Job drawing, mm, ordinate dimensions from the low corner. One solid piece. Round coordinates to 2 decimals unless told otherwise and drop trailing zeros. Loops run counter-clockwise (first coordinate to the right, second up) from the corner with the lowest first, then second, coordinate; pieces in that order, holes last. Notation, with made-up numbers: M 81,-37 L 90,-37 A19 cw 90,-3 Z; hole C -5.75,-11.75 d4. An arc over 180 degrees is marked long. Use one line per item in the form item = value.
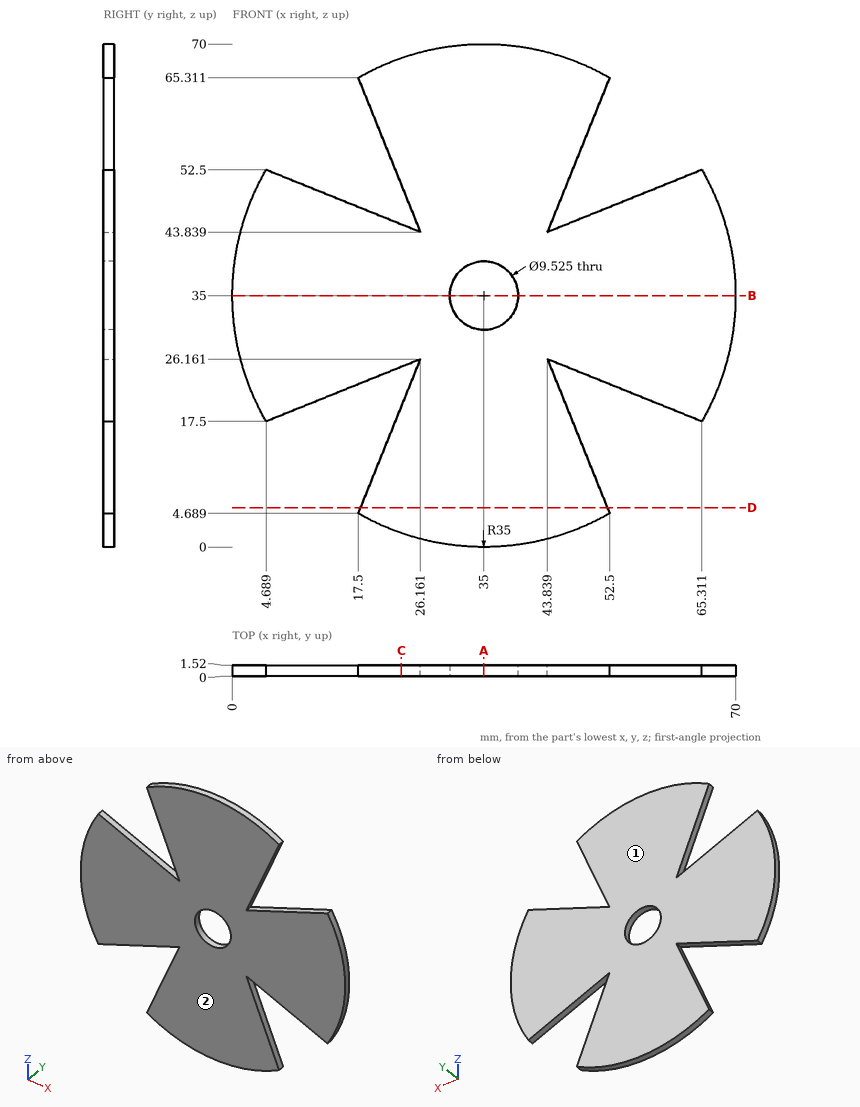
1. Probe line 1 along X through (y, z) = (0.95, 35); line 2 along X through (y, z) = (1.4, 26) (1 decimal). List the from-to ranges inside material, lowest first. Write a range as from..to.
Completed:
line_1 = 0..30.24, 39.76..70
line_2 = 1.2..25.8, 26.1..43.9, 44.2..68.8
2. Cut at A-A on x = 35. Write the cut outline in (y, z).
Completed:
outline = M 0,0 L 1.52,0 L 1.52,30.24 L 0,30.24 Z; M 0,39.76 L 1.52,39.76 L 1.52,70 L 0,70 Z
3. Pull direction Y, two halves, no side cores. Call the marked faces 1 and 2: +Y half, -Y half, draft (parallel to the pull), parting line (faces both ways), or undercut.
Completed:
face_1 = +Y half
face_2 = -Y half
4. Cut at D-D on z = 5.5. Write the cut outline in (x, y), and give its area (3 significant figures).
Completed:
outline = M 17.83,0 L 52.17,0 L 52.17,1.52 L 17.83,1.52 Z
area = 52.2 mm2
5. Drop flat-ended pins along their axis: P1, Ø4, axis at x = 29, z = 47, coming from the -Y side; P2, Ø5.5, axis at x = 35, z = 35, coming from the +Y side. Give the stop position or say it passes through.
Completed:
P1 = 0
P2 = through
6. Cut at B-B on z = 35. Write the cut outline in (x, y).
Completed:
outline = M 0,0 L 30.24,0 L 30.24,1.52 L 0,1.52 Z; M 39.76,0 L 70,0 L 70,1.52 L 39.76,1.52 Z
7. Cut at C-C on x = 23.5. Write the cut outline in (y, z).
Completed:
outline = M 0,1.94 L 1.52,1.94 L 1.52,19.56 L 0,19.56 Z; M 0,25.09 L 1.52,25.09 L 1.52,44.91 L 0,44.91 Z; M 0,50.44 L 1.52,50.44 L 1.52,68.06 L 0,68.06 Z
